Autodesk Inventor part; units mm, degrees
ref_plane "YZ Plane" through (0, 0, 0) normal (1, 0, 0) x (0, 1, 0)
ref_plane "XZ Plane" through (0, 0, 0) normal (0, 1, 0) x (-1, 0, 0)
ref_plane "XY Plane" through (0, 0, 0) normal (0, 0, 1) x (1, 0, 0)
sketch "Sketch1" plane through (0, 0, 0) normal (0, 1, 0) x (-1, 0, 0)
  circle A0 centre (0, 0) radius 5.25
  circle A1 centre (0, 0) radius 4
  dimension "d0" = 10.5
  dimension "d1" = 8
extrude "Extrusion1" add sketch "Sketch1" against normal blind 0.8 contours A0 | A1
extrude "Extrusion2" add sketch "Sketch1" along normal blind 2.7 contours A1
fillet "Fillet3" radius 0.75 1 edges at (4, 2.7, 0)
sketch "Sketch2" plane through (0, -0.8, 0) normal (0, -1, 0) x (1, 0, 0)
  arc A0 (0.4286, -2.9692) -> (2.9692, -0.4286) centre (0, 0) ccw
  line L0 (0.4286, -2.9692) -> (0.4286, -0.4286)
  arc A1 (-2.9692, -0.4286) -> (-0.4286, -2.9692) centre (0, 0) ccw
  line L1 (-0.4286, 2.9692) -> (-0.4286, 0.4286)
  arc A2 (-0.4286, 2.9692) -> (-2.9692, 0.4286) centre (0, 0) ccw
  arc A3 (2.9631, 0.4692) -> (0.4286, 2.9692) centre (0, 0) ccw
  line L2 (2.9631, 0.4692) -> (0.4286, 0.4692)
  line L3 (2.9692, -0.4286) -> (0.4286, -0.4286)
  line L4 (0.4286, 0.4692) -> (0.4286, 2.9692)
  line L5 (-0.4286, -0.4286) -> (-0.4286, -2.9692)
  line L6 (-0.4286, -0.4286) -> (-2.9692, -0.4286)
  line L7 (-0.4286, 0.4286) -> (-2.9692, 0.4286)
  circle A4 centre (0, 0) radius 3
extrude "Extrusion3" cut sketch "Sketch2" against normal blind 2 contours L0 L3 A0 | A1 L6 L5 | L2 L4 A3 | A2 L1 L7
properties part number "action-button"
The listing builds one solid part. Answer for the finished solid, in the listing's coordinates (mm). A direction names the side the tool comes from. Give positions to 0.01 mm unless a question says otherwise; leave off trailing zeros. Order: outer loops, then holes, each group sorted by start corner. A loop starts at its lowest first (then second) coordinate and runs counter-clockwise, first axis right, second up.
Item 1: The part is cut by section D-D, the plane y = 0.65. Give the vertices of the cut face in (x, z), and give its area (3 significant figures).
From the geometry:
outline: circle Ø8 at (0, 0); hole (-2.97, -0.43) arc R3 ccw to (-0.43, -2.97) - (-0.43, -0.43) - close; hole (-2.97, 0.43) - (-0.43, 0.43) - (-0.43, 2.97) arc R3 ccw to start; hole (0.43, -2.97) arc R3 ccw to (2.97, -0.43) - (0.43, -0.43) - close; hole (0.43, 0.47) - (2.96, 0.47) arc R3 ccw to (0.43, 2.97) - close
area: 31.6 mm2
Item 2: The part is cut by section C-C, the plane y = -0.4. Give the vertices of the cut face in (x, z).
From the geometry:
outline: circle Ø10.5 at (0, 0); hole (-2.97, -0.43) arc R3 ccw to (-0.43, -2.97) - (-0.43, -0.43) - close; hole (-2.97, 0.43) - (-0.43, 0.43) - (-0.43, 2.97) arc R3 ccw to start; hole (0.43, -2.97) arc R3 ccw to (2.97, -0.43) - (0.43, -0.43) - close; hole (0.43, 0.47) - (2.96, 0.47) arc R3 ccw to (0.43, 2.97) - close
Item 3: Find the intervals of material crossed by probe 1 along Z at (x, y) = (1, 1); probe 2 along X at (y, z) = (0.55, 1); probe 3 along Z at (x, y) = (-2.75, -0.05), in increasing order.
From the geometry:
probe 1: z = -3.87 to -2.83, -0.43 to 0.47, 2.83 to 3.87
probe 2: x = -3.87 to -2.83, -0.43 to 0.43, 2.83 to 3.87
probe 3: z = -4.47 to -1.2, -0.43 to 0.43, 1.2 to 4.47
Item 4: The part is cut by section A-A, the plane z = 0. Give the vertices of the cut face in (x, y), and give its area (3 significant figures).
From the geometry:
outline: (-5.25, -0.8) - (5.25, -0.8) - (5.25, 0) - (4, 0) - (4, 1.95) arc R0.75 ccw to (3.25, 2.7) - (-3.25, 2.7) arc R0.75 ccw to (-4, 1.95) - (-4, 0) - (-5.25, 0) - close
area: 29.8 mm2
Item 5: The part is cut by section B-B, the plane x = 0. Give the vertices of the cut face in (y, z).
From the geometry:
outline: (-0.8, -5.25) - (0, -5.25) - (0, -4) - (1.95, -4) arc R0.75 ccw to (2.7, -3.25) - (2.7, 3.25) arc R0.75 ccw to (1.95, 4) - (0, 4) - (0, 5.25) - (-0.8, 5.25) - close
Item 6: For a pull along X with two mould halves and no side action, classify faces 3 (the face through (0, 2.7, 0)), 4 (the face through (1, 1.2, -1)), 5 (the face through (0.867, 0.961, 3.905)) as pulls with the +X half, pulls with the -X half, needs draft (parallel to the pull), parting line crosses it, or undercut.
From the geometry:
face 3: needs draft
face 4: undercut
face 5: parting line crosses it
Item 7: Given pin 1 Ø2 at (x, y) = (-2, 0.5) entering from -Z; pin 2 Ø1.5 at (x, y) = (3.5, 1.5) entering from +Z; pin 3 Ø0.6 at (y, z) = (0.5, -1.5) entering from -X, each flat-ended and moving along its own axis, determine where each tip first touches the part or whether it passes through.
From the geometry:
pin 1: stops at z = -5.13
pin 2: stops at z = 2.9
pin 3: stops at x = -3.82
Item 8: Which of the six approach directions +Z, -Z, +X, -X, +Y, -Y give full straight-line access (tool end or side, diameter ignored) to faces 1 (the face through (0, -0.8, 0)), 2 (the face through (2, 0, 0.469))?
From the geometry:
face 1: +Z, -Z, +X, -X, -Y
face 2: -Y
